Can you work these out from the model? Positions are in its coordinate system, mm. A direction names the side the tool comes from. Round coordinates to 2 decimals unless told otherwise and drop trailing zeros. Write each loop counter-clockwise with the first axis right and the second up, starting at its lowest first coordinate (ties: lowest second). Pieces come first, ordered by that corner, then holes. Notation, with made-up numbers: M -9,86 L 37,86 A36 cw 37,122 Z; hole C 39,46.5 d5. An arc over 180 degrees is marked long. Answer in a Markdown table with one row per item. Add a question column.
(1) I'm going to push flat-ended pins straight in: pin 1 (10 mm diameter, centred on x = -4.5, y = 19.5, fed in from -Z) (3 decimals); pin 2 (2.5 mm diameter, centred on x = -15.5, z = 1.5, fed in from +Y) (3 decimals); pin 3 (1.9 mm diameter, centred on y = 10.5, z = 1, fed in from +X); pin 4 (1.5 mm diameter, centred on x = -10.5, z = -2, fed in from -Y). Where does each tip first touch, or does it pass through?
(2) Suppose I cut it at A-A, the plane y = 16. Write out the boundary of the cut face in (x, z) (3 decimals).
(3) For faces 1 (the face through (-14.05, 10, 0)), 2 (the face through (-0.56, 33.98, 2.52)), 3 (the face through (14.05, 10, 0)), which set-ups out of +Z, -Z, +X, -X, +Y, -Y let a thin tool reach every point of the face, with its end or its side?
(4) Suppose I cut it at D-D, the plane y = 31. Write out the boundary of the cut face in (x, z), then the cut area to 3 significant figures.
(5) Suppose I cut it at C-C, the plane y = 21.5. Write out the boundary of the cut face in (x, z), then the cut area to 3 significant figures.
(6) Suppose I cut it at B-B, the plane x = 16. Write out the boundary of the cut face in (y, z) (3 decimals).
(7) If I drill on probe 1 along X at (y, z) = (10, -1.75); probe 2 along Y at (x, z) = (4.5, -0.25) (3 decimals); probe 3 along X at (y, z) = (35, 0.5), over which ranges is the centre line in solid material (lowest first)?
from build123d import *

# Parameters (mm, degrees)
BOSS_EXTRUDE1_DEPTH = 19.05
SKETCH2_R           = 3.175
BOSS_EXTRUDE2_DEPTH = 50.8
BOSS_EXTRUDE2_TAPER = 1
SKETCH3_W           = 28.1
SKETCH3_H           = 13.5
BOSS_EXTRUDE3_DEPTH = 3.175


with BuildPart() as part:
    # Sketch1 → Boss-Extrude1 (new body, symmetric)
    with BuildSketch(Plane(origin=(0, 0, 0), x_dir=(0, 0, -1), z_dir=(1, 0, 0))):
        with BuildLine():
            Line((-3.175, 0), (-3.175, 3.175))
            Line((-3.175, 3.175), (3.175, 3.175))
            Line((3.175, 3.175), (3.175, 0))
            ThreePointArc((3.175, 0), (0, -3.175), (-3.175, 0))
        make_face()
    extrude(amount=BOSS_EXTRUDE1_DEPTH, both=True)

    # Sketch2 → Boss-Extrude2 (add)
    with BuildSketch(Plane(origin=(0, 0, 0), x_dir=(1, 0, 0), z_dir=(0, 1, 0))):
        Circle(SKETCH2_R)
    extrude(amount=BOSS_EXTRUDE2_DEPTH, taper=BOSS_EXTRUDE2_TAPER)

    # Sketch3 → Boss-Extrude3 (add, symmetric)
    with BuildSketch(Plane.XY):
        with Locations((0, 9.925)):
            Rectangle(SKETCH3_W, SKETCH3_H)
    extrude(amount=BOSS_EXTRUDE3_DEPTH, both=True)


solid = part.part
Calculated:
| question | item | result |
|---|---|---|
| 1 | pin 1 | z = -3.175 |
| 1 | pin 2 | y = 3.175 |
| 1 | pin 3 | x = 14.05 |
| 1 | pin 4 | y = -2.92 |
| 2 | outline | M -14.05,-3.175 L 14.05,-3.175 L 14.05,3.175 L -14.05,3.175 Z |
| 3 | face 1 | +Z, -Z, -X, +Y |
| 3 | face 2 | +Y |
| 3 | face 3 | +Z, -Z, +X, +Y |
| 4 | outline | C 0,0 d5.27 |
| 4 | area | 21.8 mm² |
| 5 | outline | C 0,0 d5.6 |
| 5 | area | 24.6 mm² |
| 6 | outline | M 0,-3.175 L 3.175,-3.175 L 3.175,3.175 L 0,3.175 A3.175 ccw Z |
| 7 | probe 1 | -14.05 to 14.05 |
| 7 | probe 2 | -3.165 to 16.675 |
| 7 | probe 3 | -2.51 to 2.51 |
